from build123d import *

# Parameters (mm, degrees)
BOX002_W     = 23
BOX002_H     = 4
BOX002_DEPTH = 1.5
BOX001_W     = 3
BOX001_H     = 36
BOX001_DEPTH = 1.5
BOX_W        = 3
BOX_H        = 36
BOX_DEPTH    = 1.5
FILLET006_R  = 0.4


with BuildPart() as cube002:
    # Box002 → Box002 (new body)
    with BuildSketch(Plane(origin=(-11.5, 18, 11.6), x_dir=(1, 0, 0), z_dir=(0, 0, 1))):
        with Locations((11.5, 2)):
            Rectangle(BOX002_W, BOX002_H)
    extrude(amount=BOX002_DEPTH)


with BuildPart() as cube001:
    # Box001 → Box001 (new body)
    with BuildSketch(Plane(origin=(8.5, -18, 11.6), x_dir=(1, 0, 0), z_dir=(0, 0, 1))):
        with Locations((1.5, 18)):
            Rectangle(BOX001_W, BOX001_H)
    extrude(amount=BOX001_DEPTH)


with BuildPart() as fillet006:
    # Box → Box (new body)
    with BuildSketch(Plane(origin=(-11.5, -18, 11.6), x_dir=(1, 0, 0), z_dir=(0, 0, 1))):
        with Locations((1.5, 18)):
            Rectangle(BOX_W, BOX_H)
    extrude(amount=BOX_DEPTH)

    # Fusion002: union Cube002, Cube001
    add(cube002.part)
    add(cube001.part)

    # Fillet006
    fillet006_edges = [fillet006.edges().sort_by_distance(p)[0] for p in [
        (-11.5, -18, 12.35),
        (-10, -18, 11.6),
        (-8.5, -18, 12.35),
        (-10, -18, 13.1),
        (10, -18, 13.1),
        (10, -18, 11.6),
        (8.5, -18, 12.35),
        (11.5, -18, 12.35),
    ]]
    fillet(fillet006_edges, radius=FILLET006_R)


solid = fillet006.part
CAD build for the part. Positions are in the model's coordinates, mm. A direction names the side the tool comes from. Round coordinates to 2 decimals unless told otherwise and drop trailing zeros. Write each loop counter-clockwise with the first axis right and the second up, starting at its lowest first coordinate (ties: lowest second). Pieces come first, ordered by that corner, then holes.
(1) Mould opens along X. For faces 3 (the face through (-8.5, 0, 12)), 4 (the face through (11.5, 2, 12)), 5 (the face through (-9, 7, 13.1)) say: pulls with the +X half, pulls with the -X half, needs draft (parallel to the pull), parting line crosses it, or undercut.
(2) Slice it at C-C, the plane x = -6.5. Write the cut outline in (y, z), and give its area (3 significant figures).
(3) Slice it at A-A, the plane y = 2. Write the cut outline in (x, z), and give its area (3 significant figures).
(4) Slice it at B-B, the plane z = 12.25. Write the cut outline in (x, y).
(5) 3-axis set-ups, long thin cutter, end or side, ignore diameter. For faces 1 (the face through (8.5, 0, 12)), 2 (the face through (-9, 7, 11.6)): which of +Z, -Z, +X, -X, +Y, -Y reach the whole face in a straight line?
(6) Probe line 1 along X through (y, z) = (-8, 13); line 2 along Y through (x, z) = (0, 12.65). List the from-to ranges inside material, lowest first.
From the geometry:
1. face 3: undercut
1. face 4: pulls with the +X half
1. face 5: needs draft
2. outline: (18, 11.6) - (22, 11.6) - (22, 13.1) - (18, 13.1) - close
2. area: 6.00 mm2
3. outline: (-11.5, 11.6) - (-8.5, 11.6) - (-8.5, 13.1) - (-11.5, 13.1) - close; (8.5, 11.6) - (11.5, 11.6) - (11.5, 13.1) - (8.5, 13.1) - close
3. area: 9.00 mm2
4. outline: (-11.5, -17.6) arc R0.4 ccw to (-11.1, -18) - (-8.9, -18) arc R0.4 ccw to (-8.5, -17.6) - (-8.5, 18) - (8.5, 18) - (8.5, -17.6) arc R0.4 ccw to (8.9, -18) - (11.1, -18) arc R0.4 ccw to (11.5, -17.6) - (11.5, 22) - (-11.5, 22) - close
5. face 1: +Z, -Z, -Y
5. face 2: -Z, +X, -X, +Y, -Y
6. line 1: x = -11.5 to -8.5, 8.5 to 11.5
6. line 2: y = 18 to 22
